```python
from build123d import *

# Parameters (mm, degrees)
BOSS_EXTRUDE1_DEPTH = 10
SKETCH2_R           = 1.5
BOSS_EXTRUDE2_DEPTH = 6
CUT_EXTRUDE1_START  = -10
SKETCH2_2_R         = 1.5
CUT_EXTRUDE1_DEPTH  = 6


with BuildPart() as part:
    # Sketch1 → Boss-Extrude1 (new body)
    with BuildSketch(Plane(origin=(0, 0, 0), x_dir=(1, 0, 0), z_dir=(0, 1, 0))):
        Polygon((1.732050808, -3), (3.464101615, 0), (1.732050808, 3), (-1.732050808, 3), (-3.464101615, 0), (-1.732050808, -3), align=None)
    extrude(amount=BOSS_EXTRUDE1_DEPTH)

    # Sketch2 → Boss-Extrude2 (add)
    with BuildSketch(Plane(origin=(0, 10, 0), x_dir=(1, 0, 0), z_dir=(0, 1, 0))):
        with Locations(Location((0, 0, 0), (0, 0, 270))):
            Circle(SKETCH2_R)
    extrude(amount=BOSS_EXTRUDE2_DEPTH)

    # Sketch2<2> → Cut-Extrude1 (cut)
    with BuildSketch(Plane(origin=(0, 10, 0), x_dir=(1, 0, 0), z_dir=(0, 1, 0)).offset(CUT_EXTRUDE1_START)):
        with Locations(Location((0, 0, 0), (0, 0, 270))):
            Circle(SKETCH2_2_R)
    extrude(amount=CUT_EXTRUDE1_DEPTH, mode=Mode.SUBTRACT)


solid = part.part
```
Work out the finished part from the listing and answer in its coordinate system (mm). A direction names the side the tool comes from. Give positions to 0.01 mm unless a question says otherwise; leave off trailing zeros. Loops run counter-clockwise (first coordinate to the right, second up) from the corner with the lowest first, then second, coordinate; pieces in that order, holes last. Notation, with made-up numbers: (76, 17.5) - (134, 17.5) arc R9 ccw to (134, 32.5) - close; hole circle Ø10 at (-29.5, -7.5). An arc over 180 degrees is marked (long way). Use CSV: the item, a comma, the result in double quotes. Start each with the question number.
(1) Find section D-D, the plane z = -2. Determine the outline of the cut face in (x, y), plus the area to 3 significant figures.
(2) Find section B-B, the plane x = 0. Determine the outline of the cut face in (y, z).
(3) Find the intervals of material crossed by L1, parallel to Y at x = 1.75, z = -2; L2, parallel to Y at x = 0.25, z = -0.5; L3, parallel to Z at x = 1.25, y = 1.25, in increasing order.
(4) A tool of negligible diameter and unlimited length cuts with its end or side. For faces 1 (the face through (1.5, 10, -0.7)), 2 (the face through (-2.6, 4.9, -1.5)), 3 (the face through (0.45, 2.96, 1.43)), from which of +Z, -Z, +X, -X, +Y, -Y can it reach the whole face along a straight path? Write none if from no direction.
(5) Determine the mould class of faces 4 (the face through (0, 6, 0)), 5 (the face through (0, 5, -3)), 6 (the face through (2.6, 4.9, 1.5)) for opening direction X: released by +X, released by -X, zero draft, split by the parting line, or undercut.
(6) Find section A-A, the plane y = 1. Determine the outline of the cut face in (x, z).
(7) This flat-tipped pin is pushed along its axis until it touches: pin 1 (0.9 mm diameter, centred on x = -0.5, z = -0.5, fed in from -Y). Where does it stop, or does it pass through?
(8) Find section C-C, the plane y = 7.75. Determine the outline of the cut face in (x, z).
Results found:
1,outline,"(-2.31, 0) - (2.31, 0) - (2.31, 10) - (-2.31, 10) - close"
1,area,"46.2 mm^2"
2,outline,"(0, -3) - (10, -3) - (10, -1.5) - (16, -1.5) - (16, 1.5) - (10, 1.5) - (10, 3) - (0, 3) - (0, 1.5) - (6, 1.5) - (6, -1.5) - (0, -1.5) - close"
3,L1,"0 to 10"
3,L2,"6 to 16"
3,L3,"-3 to -0.83, 0.83 to 3"
4,face 1,"+Y"
4,face 2,"-Z, -X, +Y, -Y"
4,face 3,"-Y"
5,face 4,"undercut"
5,face 5,"zero draft"
5,face 6,"released by +X"
6,outline,"(-3.46, 0) - (-1.73, -3) - (1.73, -3) - (3.46, 0) - (1.73, 3) - (-1.73, 3) - close; hole circle Ø3 at (0, 0)"
7,pin 1,"y = 6"
8,outline,"(-3.46, 0) - (-1.73, -3) - (1.73, -3) - (3.46, 0) - (1.73, 3) - (-1.73, 3) - close"
